Design review of the part built by this model. Coordinates are the model's own, in mm. Face numbers are marked on the shaded views. Coordinates: 2 decimals unless noted, no trailing zeros. Order: outer loops, then holes, each group sorted by start corner. A loop starts at its lowest first (then second) coordinate and runs counter-clockwise, first axis right, second up. Notation, with made-up numbers: M -29,-35.75 L 11,-35.75 A25 ccw 11,-3.75 Z; hole C 31,-17.5 d3. An arc over 180 degrees is marked long. Answer as a JSON object with one key per item and string values.
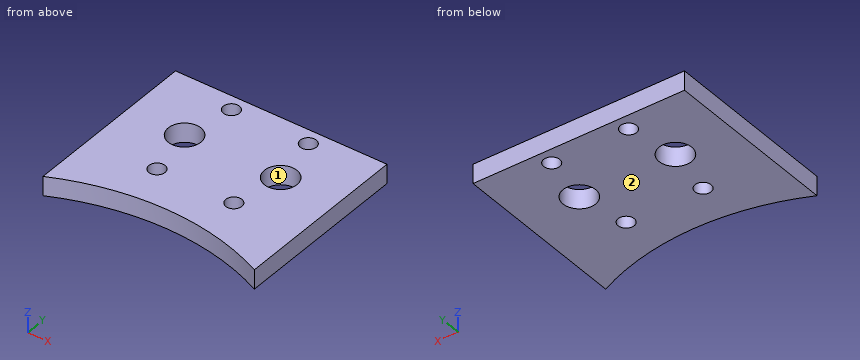
from build123d import *

# Parameters (mm, degrees)
SKETCH1_R           = 4.25
SKETCH1_R_2         = 2.1
BOSS_EXTRUDE1_DEPTH = 5
SKETCH2_W           = 23
SKETCH2_H           = 60
CUT_EXTRUDE1_DEPTH  = 10
FILLET1_R           = 5
FILLET2_R           = 5
CUT_EXTRUDE2_DEPTH  = 5


with BuildPart() as part:
    # Sketch1 → Boss-Extrude1 (new body)
    with BuildSketch(Plane.XY):
        with BuildLine():
            Line((-50.417601538, -29.831415105), (-27.417601538, -29.831415105))
            ThreePointArc((-27.417601538, -29.831415105), (0.082398462, -23.727510052), (27.582398462, -29.831415105))
            Line((27.582398462, -29.831415105), (50.582398462, -29.831415105))
            Line((50.582398462, -29.831415105), (50.582398462, 25.168584895))
            ThreePointArc((50.582398462, 25.168584895), (49.117932367, 28.704118801), (45.582398462, 30.168584895))
            Line((45.582398462, 30.168584895), (-45.417601538, 30.168584895))
            ThreePointArc((-45.417601538, 30.168584895), (-48.953135444, 28.704118801), (-50.417601538, 25.168584895))
            Line((-50.417601538, 25.168584895), (-50.417601538, -29.831415105))
        make_face()
        with Locations((12.582398462, -0.519851907)):
            Circle(SKETCH1_R, mode=Mode.SUBTRACT)
        with Locations((10.082398462, -13.519851907)):
            Circle(SKETCH1_R_2, mode=Mode.SUBTRACT)
        with Locations((-9.917601538, -13.519851907)):
            Circle(SKETCH1_R_2, mode=Mode.SUBTRACT)
        with Locations((-12.417601538, -0.519851907)):
            Circle(SKETCH1_R, mode=Mode.SUBTRACT)
        with Locations((-9.917601538, 12.480148093)):
            Circle(SKETCH1_R_2, mode=Mode.SUBTRACT)
        with Locations((10.082398462, 12.480148093)):
            Circle(SKETCH1_R_2, mode=Mode.SUBTRACT)
    extrude(amount=BOSS_EXTRUDE1_DEPTH)

    # Sketch2 → Cut-Extrude1 (cut)
    with BuildSketch(Plane.XY.offset(5)):
        with Locations((-38.917601538, 0.168584895)):
            Rectangle(SKETCH2_W, SKETCH2_H)
        with Locations((39.082398462, 0.168584895)):
            Rectangle(SKETCH2_W, SKETCH2_H)
    extrude(amount=-CUT_EXTRUDE1_DEPTH, mode=Mode.SUBTRACT)

    # Fillet1
    fillet1_edges = [part.edges().sort_by_distance(p)[0] for p in [
        (27.582398462, 30.168584895, 2.5),
    ]]
    fillet(fillet1_edges, radius=FILLET1_R)

    # Fillet2
    fillet2_edges = [part.edges().sort_by_distance(p)[0] for p in [
        (-27.417601538, 30.168584895, 2.5),
    ]]
    fillet(fillet2_edges, radius=FILLET2_R)

    # Sketch3 → Cut-Extrude2 (cut)
    with BuildSketch(Plane(origin=(0, 0, 0), x_dir=(-1, 0, 0), z_dir=(0, 0, -1))):
        with BuildLine():
            Line((-27.582398462, 25.168584895), (-27.582398462, 16.480148093))
            Line((-27.582398462, 16.480148093), (27.417601538, 16.444815638))
            Line((27.417601538, 16.444815638), (27.417601538, 25.168584895))
            ThreePointArc((27.417601538, 25.168584895), (25.953135444, 28.704118801), (22.417601538, 30.168584895))
            Line((22.417601538, 30.168584895), (-22.582398462, 30.168584895))
            ThreePointArc((-22.582398462, 30.168584895), (-26.117932367, 28.704118801), (-27.582398462, 25.168584895))
        make_face()
    extrude(amount=-CUT_EXTRUDE2_DEPTH, mode=Mode.SUBTRACT)


solid = part.part
1) Add section D-D (x = 15.5). State the section outline as (y, z) points, and give its area (3 significant figures).
Taken from the geometry:
{"outline": "M -25.58,0 L -3.61,0 L -3.61,5 L -25.58,5 Z; M 2.57,0 L 16.47,0 L 16.47,5 L 2.57,5 Z", "area": "179 mm2"}
2) Mouldability with a two-part tool opening along X and no side actions: class the marked faces 1 and 2 as released by +X, released by -X, zero draft, split by the parting line, or undercut.
Taken from the geometry:
{"face 1": "undercut", "face 2": "zero draft"}
3) Add section A-A (x = -13.5). State the section outline as (y, z) points, and give its area (3 significant figures).
Taken from the geometry:
{"outline": "M -25.16,0 L -4.63,0 L -4.63,5 L -25.16,5 Z; M 3.59,0 L 16.45,0 L 16.45,5 L 3.59,5 Z", "area": "167 mm2"}
4) To check wall thickness, follow L1, parallel to X at y = -13.5, z = 2.3; L2, parallel to Y at x = -11, z = 0.9; L3, parallel to X at y = -13, z = 2.55. State the ranges of each line that lie inside material, in increasing order.
Taken from the geometry:
{"L1": "x = -27.42 to -12.02, -7.82 to 7.98, 12.18 to 27.58", "L2": "y = -24.68 to -15.32, -11.72 to -4.53, 3.49 to 10.68, 14.28 to 16.46", "L3": "x = -27.42 to -11.95, -7.88 to 8.05, 12.12 to 27.58"}
5) Add section B-B (y = 1). State the section outline as (x, z) points.
Taken from the geometry:
{"outline": "M -27.42,0 L -16.39,0 L -16.39,5 L -27.42,5 Z; M -8.45,0 L 8.61,0 L 8.61,5 L -8.45,5 Z; M 16.55,0 L 27.58,0 L 27.58,5 L 16.55,5 Z"}
6) Add section C-C (z = 0.9). State the section outline as (x, y) points.
Taken from the geometry:
{"outline": "M -27.42,-29.83 A65 cw 27.58,-29.83 L 27.58,16.48 L -27.42,16.44 Z; hole C -12.42,-0.52 d8.5; hole C -9.92,-13.52 d4.2; hole C -9.92,12.48 d4.2; hole C 10.08,-13.52 d4.2; hole C 10.08,12.48 d4.2; hole C 12.58,-0.52 d8.5"}
